Read the model definition and answer for the solid it produces. Units are mm, in the model's axes. A direction names the side the tool comes from. Give positions to 0.01 mm unless a question says otherwise; leave off trailing zeros. Loops run counter-clockwise (first coordinate to the right, second up) from the corner with the lowest first, then second, coordinate; pieces in that order, holes last.
(1) Find section A-A, the plane x = 18. Write down the section's boundary in (y, z).
(2) Determine the mould class of faces 3 (the face through (-3, 483.5, 10)), 4 (the face through (35.052, 221, 0)), 5 (the face through (-1, 219, 12.7)) for opening direction Z: pulls with the +Z half, pulls with the -Z half, needs draft (parallel to the pull), parting line crosses it, or undercut.
(3) Find section B-B, the plane y = 210. Write down the section's boundary in (x, z).
(4) Which of the six approach directions +Z, -Z, +X, -X, +Y, -Y give full straight-line access (tool end or side, diameter ignored) to faces 1 (the face through (-1, 219, -12.7)), 2 (the face through (0, 221, -9.652))?
(5) Each of these flat-tipped pins is pushed along its axis until it touches: P1, Ø10, axis at x = -24.5, z = 0, coming from the -Y side; P2, Ø5, axis at x = -10, z = -7.5, coming from the -Y side. Where does it stop, or does it pass through?
(6) Find section C-C, the plane z = -2.25. Write down the section's boundary in (x, y).
(7) Straight lines are drawn through the part: probe 1 along Z at (x, y) = (-20, 161.5); probe 2 along X at (y, z) = (348, 6.5); probe 3 along X at (y, z) = (16, 0.25). For each, find the intervals that lie inside material, in ascending order.
```python
from build123d import *

# Parameters (mm, degrees)
SKETCH1_W               = 76.2
SKETCH1_H               = 25.4
SKETCH1_W_2             = 70.104
SKETCH1_H_2             = 19.304
BOSS_EXTRUDE1_DEPTH     = 445.4
SKETCH3_W               = 76.2
SKETCH3_H               = 25.4
SKETCH3_W_2             = 70.104
SKETCH3_H_2             = 19.304
BOSS_EXTRUDE2_DEPTH     = 38.1
SKETCH4_W               = 76.2
SKETCH4_H               = 25.4
SKETCH4_W_2             = 70.104
SKETCH4_H_2             = 19.304
BOSS_EXTRUDE3_DEPTH     = 38.1
CUT_EXTRUDE1_DEPTH      = 13.7
CUT_EXTRUDE1_DEPTH_BACK = 13.7


with BuildPart() as part:
    # Sketch1 → Boss-Extrude1 (new body)
    with BuildSketch(Plane(origin=(0, 0, 0), x_dir=(1, 0, 0), z_dir=(0, 1, 0))):
        Rectangle(SKETCH1_W, SKETCH1_H)
        Rectangle(SKETCH1_W_2, SKETCH1_H_2, mode=Mode.SUBTRACT)
    extrude(amount=BOSS_EXTRUDE1_DEPTH)

    # Sketch3 → Boss-Extrude2 (add)
    with BuildSketch(Plane.XZ):
        Rectangle(SKETCH3_W, SKETCH3_H)
        Rectangle(SKETCH3_W_2, SKETCH3_H_2, mode=Mode.SUBTRACT)
    extrude(amount=BOSS_EXTRUDE2_DEPTH)

    # Sketch4 → Boss-Extrude3 (add)
    with BuildSketch(Plane(origin=(0, 445.4, 0), x_dir=(1, 0, 0), z_dir=(0, 1, 0))):
        Rectangle(SKETCH4_W, SKETCH4_H)
        Rectangle(SKETCH4_W_2, SKETCH4_H_2, mode=Mode.SUBTRACT)
    extrude(amount=BOSS_EXTRUDE3_DEPTH)

    # Sketch5 → Cut-Extrude1 (cut, two sides)
    with BuildSketch(Plane(origin=(-500, 0, 0), x_dir=(1, 0, 0), z_dir=(0, 0, -1))) as cut_extrude1_sk:
        Polygon((607.156068895, 107.156068895), (437.011376746, -62.988623254), (437.011376746, 107.156068895), align=None)
    extrude(amount=CUT_EXTRUDE1_DEPTH, mode=Mode.SUBTRACT)
    extrude(cut_extrude1_sk.sketch, amount=-CUT_EXTRUDE1_DEPTH_BACK, mode=Mode.SUBTRACT)


solid = part.part
```
Entries:
1. outline: (-18, -12.7) - (483.5, -12.7) - (483.5, -9.65) - (-18, -9.65) - close; (-18, 9.65) - (483.5, 9.65) - (483.5, 12.7) - (-18, 12.7) - close
2. face 3: needs draft
2. face 4: undercut
2. face 5: pulls with the +Z half
3. outline: (-38.1, -12.7) - (38.1, -12.7) - (38.1, 12.7) - (-38.1, 12.7) - close; hole (-35.05, -9.65) - (35.05, -9.65) - (35.05, 9.65) - (-35.05, 9.65) - close
4. face 1: -Z, +X, -X, +Y, -Y
4. face 2: +Y, -Y
5. P1: passes through
5. P2: stops at y = 8.73
6. outline: (-38.1, 38.1) - (-35.05, 35.05) - (-35.05, 483.5) - (-38.1, 483.5) - close; (35.05, -35.05) - (38.1, -38.1) - (38.1, 483.5) - (35.05, 483.5) - close
7. probe 1: z = -12.7 to -9.65, 9.65 to 12.7
7. probe 2: x = -38.1 to -35.05, 35.05 to 38.1
7. probe 3: x = 35.05 to 38.1
